Source: three-view drawing plus pictorial views. Frame: mm from the lowest corner of the part. A direction names the side the tool comes from. Give positions to 0.01 mm unless a question says otherwise; leave off trailing zeros. Order: outer loops, then holes, each group sorted by start corner. A loop starts at its lowest first (then second) coordinate and runs counter-clockwise, first axis right, second up. Notation, with made-up numbers: (-17, 70) -> (36, 70) arc R19 cw to (36, 100) -> close; hole circle Ø2 at (56, 27.5). An arc over 180 degrees is marked (long way). One line per question, with ' | ' between items.
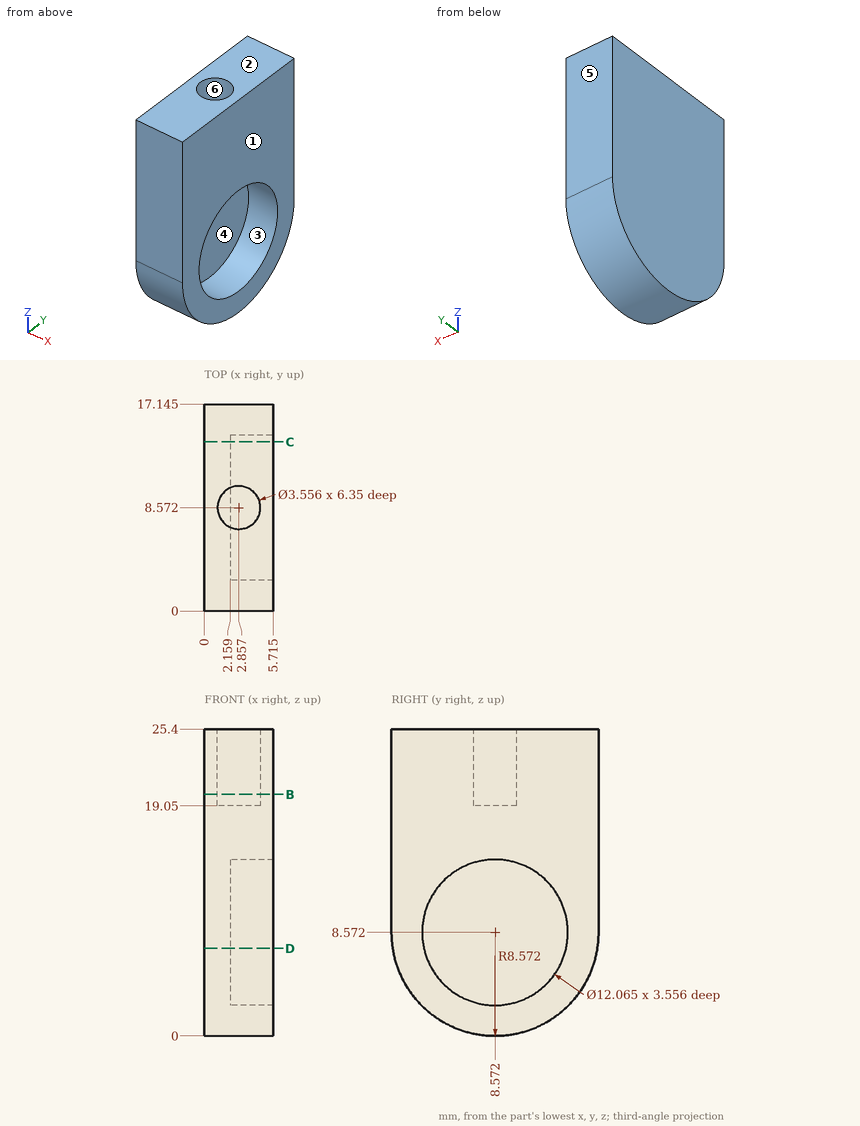
1) Set-up query: the marked faces 4, 5 and 6. Return all of +Z, -Z, +X, -X, +Y, -Y with unobstructed straight access to the full face (end or side cutting, diameter ignored); none if empty.
Check result:
face 4: +X | face 5: +Z, -Z, +X, -X, +Y | face 6: +Z
2) Material intervals for probe 1 along X at (y, z) = (11.5, 3.75); probe 2 along Z at (x, y) = (4.6, 10) (1 decimal); probe 3 along Z at (x, y) = (3.5, 10.5) (1 decimal), sorted ascending. Write a range as from..to.
Check result:
probe 1: x = 0..2.16 | probe 2: z = 0.1..2.7, 14.4..25.4 | probe 3: z = 0.2..2.9, 14.3..25.4
3) Section C-C on y = 14. Return loops of the section in (x, z) (1 decimal).
Check result:
outline: (0, 1.9) -> (5.7, 1.9) -> (5.7, 5.9) -> (2.2, 5.9) -> (2.2, 11.2) -> (5.7, 11.2) -> (5.7, 25.4) -> (0, 25.4) -> close
4) Pull-direction query (Z, two-part tool) for the marked faces 1, 2 and 3; classes: +Z half, -Z half, draft (parallel to the pull), parting line (faces both ways), or undercut.
Check result:
face 1: draft | face 2: +Z half | face 3: undercut
5) Contact query for a flat-ended pin moving along its axis: pin 1 Ø3.5 at (y, z) = (7, 11.5) entering from +X. Output: stop coordinate, or through.
Check result:
pin 1: stops at x = 2.16
6) Section B-B on z = 20. Return loops of the section in (x, y) (1 decimal).
Check result:
outline: (0, 0) -> (5.7, 0) -> (5.7, 17.1) -> (0, 17.1) -> close; hole circle Ø3.6 at (2.9, 8.6)
7) Section D-D on z = 7.25. Return loops of the section in (x, y) (1 decimal).
Check result:
outline: (0, 0.1) -> (5.7, 0.1) -> (5.7, 2.7) -> (2.2, 2.7) -> (2.2, 14.5) -> (5.7, 14.5) -> (5.7, 17) -> (0, 17) -> close
